Autodesk Inventor part; units mm, degrees
ref_plane "YZ Plane" through (0, 0, 0) normal (1, 0, 0) x (0, 1, 0)
ref_plane "XZ Plane" through (0, 0, 0) normal (0, 1, 0) x (-1, 0, 0)
ref_plane "XY Plane" through (0, 0, 0) normal (0, 0, 1) x (1, 0, 0)
sketch "Sketch1" plane through (0, 0, 0) normal (0, 1, 0) x (-1, 0, 0)
  line L0 (0, 0) -> (70, 0)
  line L1 (70, 0) -> (70, -55)
  line L2 (70, -55) -> (0, -55)
  line L3 (0, -55) -> (0, 0)
  line L4 (51.25, -32.75) -> (40.75, -32.75)
  line L5 (40.75, -32.75) -> (40.75, -22.25)
  line L6 (40.75, -22.25) -> (51.25, -22.25)
  line L7 (51.25, -22.25) -> (51.25, -32.75)
  line L8 (26, -48.75) -> (8, -48.75)
  line L9 (8, -48.75) -> (8, -6.25)
  line L10 (8, -6.25) -> (26, -6.25)
  line L11 (26, -6.25) -> (26, -48.75)
  dimension "d0" = 70
  dimension "d1" = 55
  dimension "d2" = 10.5
  dimension "d3" = 10.5
  dimension "d4" = 18
  dimension "d5" = 42.5
  dimension "d6" = 6.25
  dimension "d7" = 22.25
  dimension "d8" = 8
  dimension "d9" = 18.75
extrude "Extrusion1" add sketch "Sketch1" along normal blind 4
sketch "Sketch2" plane through (0, 0, 0) normal (0, -1, 0) x (1, 0, 0)
  line L0 (0, 0) -> (0, -55)
  line L1 (-70, 0) -> (0, 0)
  line L2 (0, -55) -> (-70, -55)
  line L3 (-70, -55) -> (-70, 0)
  line L4 (-70, 0) -> (0, 0)
  line L5 (0, 0) -> (0, -55)
  line L6 (-3, -52) -> (-67, -52)
  line L7 (-67, -52) -> (-67, -3)
  line L8 (-67, -3) -> (-3, -3)
  line L9 (-3, -3) -> (-3, -52)
  line L10 (-29.5, -43.75) -> (-62.25, -43.75)
  line L11 (-62.25, -43.75) -> (-62.25, -11.25)
  line L12 (-62.25, -11.25) -> (-29.5, -11.25)
  line L13 (-40.75, -32.75) -> (-51.25, -32.75)
  line L14 (-51.25, -22.25) -> (-40.75, -22.25)
  line L15 (-51.25, -32.75) -> (-51.25, -22.25)
  line L16 (-40.75, -22.25) -> (-40.75, -32.75)
  line L17 (-29.5, -45.75) -> (-64.25, -45.75)
  line L18 (-64.25, -45.75) -> (-64.25, -9.25)
  line L19 (-64.25, -9.25) -> (-29.5, -9.25)
  line L20 (-29.5, -45.75) -> (-29.5, -43.75)
  line L21 (-29.5, -11.25) -> (-29.5, -9.25)
  dimension "d14" = 3
  dimension "d15" = 3
  dimension "d16" = 3
  dimension "d17" = 3
  dimension "d18" = 32.75
  dimension "d19" = 11
  dimension "d20" = 11
  dimension "d21" = 11
  dimension "d23" = 2
  dimension "d24" = 2
  dimension "d25" = 2
extrude "Extrusion2" add sketch "Sketch2" along normal blind 3 contours L20 L17 L18 L19 L21 L12 L11 L10
sketch "Sketch3" plane through (0, 0, 0) normal (0, -1, 0) x (1, 0, 0)
  line L0 (0, -55) -> (0, 0)
  line L1 (0, -55) -> (-70, -55)
  line L2 (-70, -55) -> (-70, 0)
  line L3 (-70, 0) -> (0, 0)
  line L4 (0, 0) -> (0, -55)
  line L5 (-3, -52) -> (-67, -52)
  line L6 (-67, -52) -> (-67, -3)
  line L7 (-67, -3) -> (-3, -3)
  line L8 (-3, -3) -> (-3, -52)
  dimension "d28" = 3
  dimension "d29" = 3
  dimension "d30" = 3
  dimension "d31" = 3
extrude "Extrusion3" add sketch "Sketch3" along normal blind 31
properties part number "test_camAndultra"
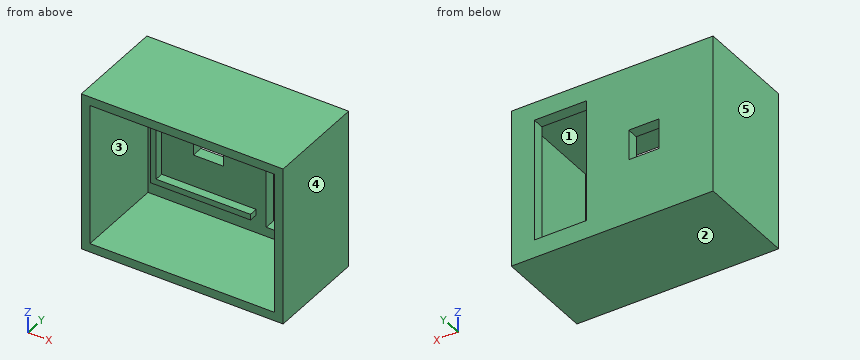
Geometry check sheet. Reference: the model listing, model coordinates, mm. Face numbers are marked on the shaded views. A direction names the side the tool comes from. Round coordinates to 2 decimals unless told otherwise and drop trailing zeros. Order: outer loops, then holes, each group sorted by start corner. A loop starts at its lowest first (then second) coordinate and runs counter-clockwise, first axis right, second up. Notation, with made-up numbers: (69, 54) - (105, 54) arc R7 cw to (105, 63) - close; hole circle Ø3 at (23.25, 29). An arc over 180 degrees is marked (long way). Use a Markdown table: item, result. Add a question column.
1) Section check B-B (x = -19.5). Record the cut outline in (y, z).
2) Section check C-C (y = -25). Record the cut outline in (x, z).
3) Section check A-A (z = -31.5). Record the cut outline in (x, y), then the cut area to 3 significant figures.
4) Set-up check for the marked faces 1 and 2: record each of +Z, -Z, +X, -X, +Y, -Y from which the full face is reachable in a straight line by a thin tool's end or side.
5) Section check D-D (x = -46). Record the cut outline in (y, z), then the cut area to 3 significant figures.
6) Mould release check, pull along X, two halves, no side actions. Record for the marked faces 3, 4 and 5: released by +X, released by -X, zero draft, split by the parting line, or undercut.
7) Gauge pin test, flat end, axial feed: P1, Ø1, axis at x = -36.5, z = -16, coming from the -Y side. Record the tip position at first contact, or that the pin passes through.
8) Thickness scan on line 1 along X through (y, z) = (-2.5, -11.5); line 2 along X through (y, z) = (1, -40.5); line 3 along Z through (x, y) = (-23, -22.5). Record the ranges inside material, lowest first.
Established:
| question | item | result |
|---|---|---|
| 1 | outline | (-31, -55) - (4, -55) - (4, -48.75) - (0, -48.75) - (0, -52) - (-31, -52) - close; (-31, -3) - (0, -3) - (0, -6.25) - (4, -6.25) - (4, 0) - (-31, 0) - close |
| 2 | outline | (-70, -55) - (0, -55) - (0, 0) - (-70, 0) - close; hole (-67, -52) - (-3, -52) - (-3, -3) - (-67, -3) - close |
| 3 | outline | (-70, -31) - (-67, -31) - (-67, 0) - (-64.25, 0) - (-64.25, -3) - (-62.25, -3) - (-62.25, 0) - (-51.25, 0) - (-51.25, 4) - (-70, 4) - close; (-40.75, 0) - (-26, 0) - (-26, 4) - (-40.75, 4) - close; (-8, 0) - (-3, 0) - (-3, -31) - (0, -31) - (0, 4) - (-8, 4) - close |
| 3 | area | 358 mm2 |
| 4 | face 1 | -Y |
| 4 | face 2 | -Z, +X, -X, +Y, -Y |
| 5 | outline | (-31, -55) - (4, -55) - (4, -32.75) - (0, -32.75) - (0, -43.75) - (-3, -43.75) - (-3, -45.75) - (0, -45.75) - (0, -52) - (-31, -52) - close; (-31, -3) - (0, -3) - (0, -9.25) - (-3, -9.25) - (-3, -11.25) - (0, -11.25) - (0, -22.25) - (4, -22.25) - (4, 0) - (-31, 0) - close |
| 5 | area | 376 mm2 |
| 6 | face 3 | undercut |
| 6 | face 4 | released by +X |
| 6 | face 5 | released by -X |
| 7 | P1 | y = 0 |
| 8 | line 1 | -70 to -67, -64.25 to -62.25, -3 to 0 |
| 8 | line 2 | -70 to -26, -8 to 0 |
| 8 | line 3 | -55 to -52, -3 to 0 |
